```python
from build123d import *

# Parameters (mm, degrees)
F1_DEPTH = 7


with BuildPart() as f1:
    # F0 (on Front) → F1 (new body)
    with BuildSketch(Plane.XZ):
        Polygon((-8.290611, 55.949569), (-14.560611, 55.949569), (-14.560611, 26.091313), (-15.139798, 25.439247), (-33.160611, 25.439247), (-33.160611, 6.169569), (-8.290611, 6.169569), (-8.290611, 16.149569), (-14.260611, 16.149569), (-14.260611, 15.149569), (-17.360611, 15.149569), (-17.360611, 16.149569), (-24.360611, 16.149569), (-24.360611, 18.949569), (-17.360611, 18.949569), (-17.360611, 20.439569), (-14.260611, 20.439569), (-14.260611, 19.149569), (-8.290611, 19.149569), (-8.290611, 29.249569), (-1.160611, 29.249569), (-1.160611, 44.349569), (-8.290611, 44.349569), align=None)
    extrude(amount=F1_DEPTH)


solid = f1.part
```
For this review, take the finished solid that the model builds, in its own axes (mm). A direction names the side the tool comes from. Give positions to 0.01 mm unless a question says otherwise; leave off trailing zeros. Write each loop counter-clockwise with the first axis right and the second up, starting at its lowest first coordinate (ties: lowest second). Pieces come first, ordered by that corner, then holes. Notation, with made-up numbers: M -24.5,20.25 L 1.5,20.25 A30 cw 1.5,51.25 Z; hole C 33.5,23 d11. An arc over 180 degrees is marked long. One line per item, written item: value.
1) The part is to be moulded in two halves that separate along Z. For faces 4 (the flat face through (-17.361, -3, 20)), 5 (the flat face through (-8.291, -3, 11)), 6 (the flat face through (-21, -3, 6.17)), 7 (the flat face through (-14.261, -3.5, 15.7)), say which applies: +Z half, -Z half, draft (parallel to the pull), parting line (faces both ways), or undercut.
Results are:
face 4: undercut
face 5: draft
face 6: -Z half
face 7: undercut
2) For P1, Ø1.1, axis at y = -2.5, z = 15.5, coming from the +X side; P2, Ø3.5, axis at x = -5.5, y = -4.5, coming from the +Z side, all flat-tipped, find the tip position at first contact; note any pin that passes through.
Results are:
P1: stops at x = -8.29
P2: stops at z = 44.35
3) Take a section at B-B, the plane y = -0.75. Write out the cut boundary in (x, z).
Results are:
outline: M -33.16,6.17 L -8.29,6.17 L -8.29,16.15 L -14.26,16.15 L -14.26,15.15 L -17.36,15.15 L -17.36,16.15 L -24.36,16.15 L -24.36,18.95 L -17.36,18.95 L -17.36,20.44 L -14.26,20.44 L -14.26,19.15 L -8.29,19.15 L -8.29,29.25 L -1.16,29.25 L -1.16,44.35 L -8.29,44.35 L -8.29,55.95 L -14.56,55.95 L -14.56,26.09 L -15.14,25.44 L -33.16,25.44 Z
4) Take a section at D-D, the plane z = 32.5. Write out the cut boundary in (x, y), then the cut area to 3 significant figures.
Results are:
outline: M -14.56,-7 L -1.16,-7 L -1.16,0 L -14.56,0 Z
area: 93.8 mm²
5) Take a section at C-C, the plane x = -13.5. Write out the cut boundary in (y, z), then the cut area to 3 significant figures.
Results are:
outline: M -7,6.17 L 0,6.17 L 0,16.15 L -7,16.15 Z; M -7,19.15 L 0,19.15 L 0,55.95 L -7,55.95 Z
area: 327 mm²
6) Take a section at A-A, the plane x = -19.5. Write out the cut boundary in (y, z).
Results are:
outline: M -7,6.17 L 0,6.17 L 0,16.15 L -7,16.15 Z; M -7,18.95 L 0,18.95 L 0,25.44 L -7,25.44 Z
7) For faces 1 (the flat face through (-5, -3, 44.35)), 2 (the flat face through (-17.361, -3.5, 15.6)), 3 (the flat face through (-14.561, -3, 41)), list the 3-axis set-ups (+Z, -Z, +X, -X, +Y, -Y) from which the entire face can be reached by the end or side of a thin tool; tool diameter is ignored.
Results are:
face 1: +Z, +X, +Y, -Y
face 2: +Y, -Y
face 3: +Z, -X, +Y, -Y
8) For line 1 (Z direction, x = -17.5, y = -4.5); line 2 (Z direction, x = -10, y = -4); line 3 (X direction, y = -3.5, z = 44), list the stretches that pass through material, from the lowest coordinate up. Write a range as from..to.
Results are:
line 1: z = 6.17..16.15, 18.95..25.44
line 2: z = 6.17..16.15, 19.15..55.95
line 3: x = -14.56..-1.16
